```python
from build123d import *

# Parameters (mm, degrees)
BOSS_EXTRUDE1_DEPTH                          = 5
FILLET1_R                                    = 10
CBORE_FOR_M3_HEX_SOCKET_HEAD_CAP_SCR_2_COUNT = 2
CBORE_FOR_M3_HEX_SOCKET_HEAD_CAP_SCR_2_PITCH = 90
M2_5_TAPPED_HOLE1_D                          = 2.05
M2_5_TAPPED_HOLE1_DEPTH                      = 6.35
M2_5_TAPPED_HOLE1_TIP                        = 0.615882135


with BuildPart() as part:
    # Sketch1 → Boss-Extrude1 (new body)
    with BuildSketch(Plane.XY):
        with BuildLine():
            Line((0, 11), (0, 14))
            Line((0, 14), (-14, 14))
            Line((-14, 14), (-46.365742902, 4.809859283))
            ThreePointArc((-46.365742902, 4.809859283), (-48.989280293, 3.014239995), (-50, 0))
            Line((-50, 0), (-45, 0))
            Line((-45, 0), (-11, 0))
            ThreePointArc((-11, 0), (-7.778174593, 7.778174593), (0, 11))
        make_face()
    extrude(amount=BOSS_EXTRUDE1_DEPTH)

    # Fillet1
    fillet1_edges = [part.edges().sort_by_distance(p)[0] for p in [
        (-14, 14, 2.5),
    ]]
    fillet(fillet1_edges, radius=FILLET1_R)

    # Mirror1: part across plane


with BuildPart() as part_1:
    add(part.part)
    add(part.part.mirror(Plane(origin=(-45, 0, 5), x_dir=(0, 0, 1), z_dir=(0, -1, 0))))

    # Mirror2: part across plane


with BuildPart() as part_2:
    add(part_1.part)
    add(part_1.part.mirror(Plane(origin=(0, -11, 5), x_dir=(0, 0, 1), z_dir=(-1, 0, 0))))

    # Sketch4 → CBORE for M3 Hex Socket Head Cap Screw1 (revolve, cut)
    with BuildSketch(Plane(origin=(-45, 0, 5), x_dir=(0, -1, 0), z_dir=(1, 0, 0))):
        Polygon((0, 0), (0, 12.521463052), (1.7, 11.5), (1.7, 3.4), (3.25, 3.4), (3.25, 0.025), (3.275, 0), align=None)
    cbore_for_m3_hex_socket_head_cap_screw1 = revolve(axis=Axis((-45, 0, 11.35), (0, 0, -1)), mode=Mode.SUBTRACT)

    # CBORE for M3 Hex Socket Head Cap Scr 2: CBORE for M3 Hex Socket Head Cap Screw1 ×2
    with Locations(*[(i * CBORE_FOR_M3_HEX_SOCKET_HEAD_CAP_SCR_2_PITCH, 0, 0) for i in range(1, CBORE_FOR_M3_HEX_SOCKET_HEAD_CAP_SCR_2_COUNT)]):
        add(cbore_for_m3_hex_socket_head_cap_screw1, mode=Mode.SUBTRACT)

    # M2.5 Tapped Hole1
    with Locations(Plane.XY.offset(5)):
        with Locations((-11.5, 11.5), (11.5, 11.5), (11.5, -11.5), (-11.5, -11.5)):
            Hole(M2_5_TAPPED_HOLE1_D / 2, depth=M2_5_TAPPED_HOLE1_DEPTH)
            with Locations((0, 0, -(M2_5_TAPPED_HOLE1_DEPTH + M2_5_TAPPED_HOLE1_TIP / 2))):  # 118° drill point
                Cone(0, M2_5_TAPPED_HOLE1_D / 2, M2_5_TAPPED_HOLE1_TIP, mode=Mode.SUBTRACT)


solid = part_2.part
```
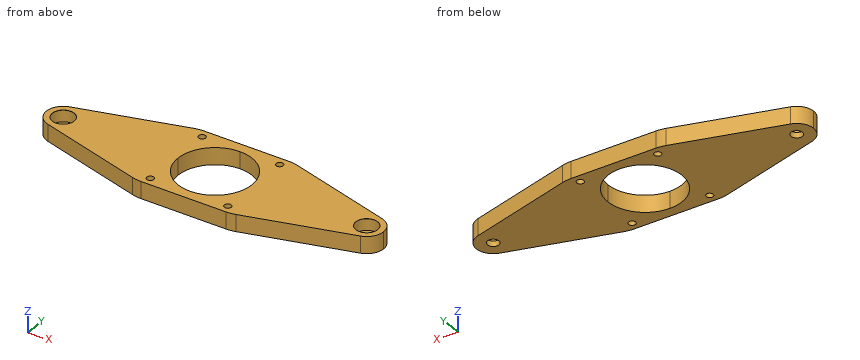
Build history of the part. All positions in model axes, mm. Round coordinates to 2 decimals unless told otherwise and drop trailing zeros. Order: outer loops, then holes, each group sorted by start corner. A loop starts at its lowest first (then second) coordinate and runs counter-clockwise, first axis right, second up. Notation, with made-up numbers: (42.5, 4) -> (49.5, 4) arc R21 cw to (49.5, 15) -> close; hole circle Ø7 at (-11, 3.5). An arc over 180 degrees is marked (long way). Answer in a Markdown table with one row per item.
1) Band-saw the part on B-B on x = 7.5. Give the cut face in (y, z), and give its area (3 significant figures).
Values:
| item | result |
|---|---|
| outline | (-14, 0) -> (-8.05, 0) -> (-8.05, 5) -> (-14, 5) -> close; (8.05, 0) -> (14, 0) -> (14, 5) -> (8.05, 5) -> close |
| area | 59.5 mm2 |
2) Wall check: L1, parallel to Y at x = -11.5, z = 2.05 (3 decimals); L2, parallel to X at y = 0, z = 2.8; L3, parallel to X at y = 1.5, z = 2.2. Give the ranges that are in metal, low to high.
Values:
| item | result |
|---|---|
| L1 | -14 to -12.525, -10.475 to 10.475, 12.525 to 14 |
| L2 | -50 to -48.25, -41.75 to -11, 11 to 41.75, 48.25 to 50 |
| L3 | -49.77 to -47.88, -42.12 to -10.9, 10.9 to 42.12, 47.88 to 49.77 |
3) Band-saw the part on C-C on y = -7. Give the cut face in (x, z), and give its area (3 significant figures).
Values:
| item | result |
|---|---|
| outline | (-38.65, 0) -> (-8.49, 0) -> (-8.49, 5) -> (-38.65, 5) -> close; (8.49, 0) -> (38.65, 0) -> (38.65, 5) -> (8.49, 5) -> close |
| area | 302 mm2 |
4) Band-saw the part on D-D on x = 45. Give the cut face in (y, z) (3 decimals), and give its area (3 significant figures).
Values:
| item | result |
|---|---|
| outline | (-5.198, 0) -> (-1.7, 0) -> (-1.7, 1.6) -> (-3.25, 1.6) -> (-3.25, 4.975) -> (-3.275, 5) -> (-5.198, 5) -> close; (1.7, 0) -> (5.198, 0) -> (5.198, 5) -> (3.275, 5) -> (3.25, 4.975) -> (3.25, 1.6) -> (1.7, 1.6) -> close |
| area | 24.4 mm2 |
5) Band-saw the part on A-A on z = 2.5. Give the cut face in (x, y) (3 decimals), and give its area (3 significant figures).
Values:
| item | result |
|---|---|
| outline | (-46.366, -4.81) -> (-15.339, -13.62) arc R10 ccw to (-12.608, -14) -> (12.608, -14) arc R10 ccw to (15.339, -13.62) -> (46.366, -4.81) arc R5 ccw to (46.366, 4.81) -> (15.339, 13.62) arc R10 ccw to (12.608, 14) -> (-12.608, 14) arc R10 ccw to (-15.339, 13.62) -> (-46.366, 4.81) arc R5 ccw to start; hole circle Ø6.5 at (-45, 0); hole circle Ø2.05 at (-11.5, -11.5); hole circle Ø2.05 at (-11.5, 11.5); hole circle Ø22 at (0, 0); hole circle Ø2.05 at (11.5, -11.5); hole circle Ø2.05 at (11.5, 11.5); hole circle Ø6.5 at (45, 0) |
| area | 1,590 mm2 |
6) Pin check, flat tips, straight feed: P1, Ø10.5, axis at x = -45, y = 0, coming from the +Z side; P2, Ø2, axis at x = 15.5, z = 4, coming from the -Y side; P3, Ø5.5, axis at x = 45, y = 0, coming from the +Z side. Stop position of each tip, or through.
Values:
| item | result |
|---|---|
| P1 | z = 5 |
| P2 | y = -13.82 |
| P3 | z = 1.6 |
